Build history of the part. All positions in model axes, mm. Face numbers are marked on the shaded views. A direction names the side the tool comes from. Give positions to 0.01 mm unless a question says otherwise; leave off trailing zeros. Loops run counter-clockwise (first coordinate to the right, second up) from the corner with the lowest first, then second, coordinate; pieces in that order, holes last. Notation, with made-up numbers: M -32,57 L -1,57 A18 cw -1,74 Z; hole C -4.75,49 d8. An arc over 180 degrees is marked long. Put each result on its own line as item: value.
```python
from build123d import *

# Parameters (mm, degrees)
SKETCH1_R           = 45
BOSS_EXTRUDE1_DEPTH = 8
SKETCH2_R           = 35.05
CUT_EXTRUDE1_DEPTH  = 4
SKETCH3_R           = 20
SKETCH3_W           = 14.2
SKETCH3_H           = 14.2
BOSS_EXTRUDE2_DEPTH = 13
CHAMFER1_SIZE       = 0.5
BOSS_EXTRUDE3_DEPTH = 14
CHAMFER3_SIZE       = 1
FILLET1_R           = 1


with BuildPart() as part:
    # Sketch1 → Boss-Extrude1 (new body)
    with BuildSketch(Plane.XY):
        Circle(SKETCH1_R)
    extrude(amount=BOSS_EXTRUDE1_DEPTH)

    # Sketch2 → Cut-Extrude1 (cut)
    with BuildSketch(Plane.XY.offset(8)):
        Circle(SKETCH2_R)
    extrude(amount=-CUT_EXTRUDE1_DEPTH, mode=Mode.SUBTRACT)

    # Sketch3 → Boss-Extrude2 (add)
    with BuildSketch(Plane.XY.offset(4)):
        with Locations(Location((0, 0, 0), (0, 0, 180))):
            Circle(SKETCH3_R)
        Rectangle(SKETCH3_W, SKETCH3_H, mode=Mode.SUBTRACT)
    extrude(amount=BOSS_EXTRUDE2_DEPTH)

    # Chamfer1
    chamfer1_edges = [part.edges().sort_by_distance(p)[0] for p in [
        (20, 0, 17),
        (-7.1, 0, 17),
        (0, -7.1, 17),
        (7.1, 0, 17),
        (0, 7.1, 17),
        (-45, 0, 8),
        (-35.05, 0, 8),
    ]]
    chamfer(chamfer1_edges, length=CHAMFER1_SIZE)

    # Sketch4 → Boss-Extrude3 (add)
    with BuildSketch(Plane(origin=(0, 0, 0), x_dir=(-1, 0, 0), z_dir=(0, 0, -1))):
        Polygon((-2.5, 2.5), (-37.5, 2.5), (-37.5, -2.5), (-2.5, -2.5), (-2.5, -37.5), (2.5, -37.5), (2.5, -2.5), (37.5, -2.5), (37.5, 2.5), (2.5, 2.5), (2.5, 37.5), (-2.5, 37.5), align=None)
    extrude(amount=BOSS_EXTRUDE3_DEPTH)

    # Chamfer3
    chamfer3_edges = [part.edges().sort_by_distance(p)[0] for p in [
        (0, 37.5, -14),
        (37.5, 0, -14),
        (0, -37.5, -14),
        (-37.5, 0, -14),
    ]]
    chamfer(chamfer3_edges, length=CHAMFER3_SIZE)

    # Fillet1
    fillet1_edges = [part.edges().sort_by_distance(p)[0] for p in [
        (-2.5, 2.5, -7),
        (2.5, 2.5, -7),
        (2.5, -2.5, -7),
        (-2.5, -2.5, -7),
    ]]
    fillet(fillet1_edges, radius=FILLET1_R)


solid = part.part
```
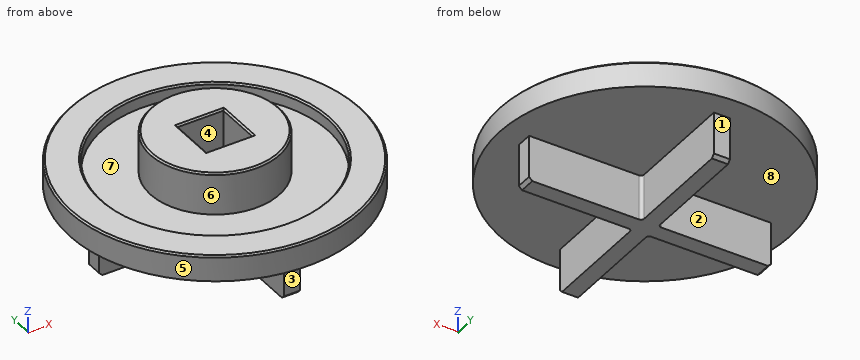
Q1. Slice it at C-C (z = -6). List the corners of the cut face in (x, y).
Here are the results:
outline: M -37.5,-2.5 L -3.5,-2.5 A1 cw -2.5,-3.5 L -2.5,-37.5 L 2.5,-37.5 L 2.5,-3.5 A1 cw 3.5,-2.5 L 37.5,-2.5 L 37.5,2.5 L 3.5,2.5 A1 cw 2.5,3.5 L 2.5,37.5 L -2.5,37.5 L -2.5,3.5 A1 cw -3.5,2.5 L -37.5,2.5 Z
Q2. Probe line 1 (Y direction, x = 0, z = 6.4); line 2 (X direction, y = 18.5, z = -8.5); line 3 (Z direction, x = -27.5, y = 9.5). List the from-to ranges inside material, lowest first. Write a range as from..to.
Here are the results:
line 1: -45..-35.05, -20..-7.1, 7.1..20, 35.05..45
line 2: -2.5..2.5
line 3: 0..4
Q3. Drop flat-ended pins along their axis: pin 1 Ø2.5 at (y, z) = (0, -6) entering from +X; pin 2 Ø8 at (x, z) = (30, -9.5) entering from +Y; pin 3 Ø4 at (y, z) = (-27.5, -7) entering from -X. Give the stop position or say it passes through.
Here are the results:
pin 1: x = 37.5
pin 2: y = 2.5
pin 3: x = -2.5
Q4. Mould opens along Y. For the marked faces 5, 6, 7 and 8 say: pulls with the +Y half, pulls with the -Y half, needs draft (parallel to the pull), parting line crosses it, or undercut.
Here are the results:
face 5: parting line crosses it
face 6: undercut
face 7: undercut
face 8: needs draft
Q5. Tool access for the marked faces 1, 2, 3 and 4: list every direction of +Z, -Z, +X, -X, +Y, -Y with a clear straight run to the whole face (end or side of a thin tool).
Here are the results:
face 1: -Z, +X, -X, +Y
face 2: -Z, -X, +Y
face 3: -Z, +X, -X, -Y
face 4: +Z
